Work out the finished part from the listing and answer in its coordinate system (mm). Round coordinates to 2 decimals unless told otherwise and drop trailing zeros. Order: outer loops, then holes, each group sorted by start corner. A loop starts at its lowest first (then second) coordinate and runs counter-clockwise, first axis right, second up. Notation, with made-up numbers: (21, 55) -> (43, 55) arc R22 ccw to (43, 72) -> close; hole circle Ø3 at (43.5, -2.5). An arc over 180 degrees is marked (long way). Use one line per item in the form item = value.
```python
from build123d import *

# Parameters (mm, degrees)
BOSS_EXTRUDE1_DEPTH = 3
FILLET1_R           = 10
SKETCH2_R           = 4.25
CUT_EXTRUDE1_DEPTH  = 126.335549626


with BuildPart() as part:
    # Sketch1 → Boss-Extrude1 (new body)
    with BuildSketch(Plane.XY):
        Polygon((0, 0), (0, 60), (110, 60), (110, 20), (75.358983849, 0), align=None)
    extrude(amount=BOSS_EXTRUDE1_DEPTH)

    # Fillet1
    fillet1_edges = [part.edges().sort_by_distance(p)[0] for p in [
        (110, 60, 1.5),
        (110, 20, 1.5),
        (75.358983849, 0, 1.5),
    ]]
    fillet(fillet1_edges, radius=FILLET1_R)

    # Sketch2 → Cut-Extrude1 (cut, through all)
    with BuildSketch(Plane.XY.offset(3)):
        with Locations((35, 15)):
            Circle(SKETCH2_R)
        with Locations((85, 45)):
            Circle(SKETCH2_R)
    extrude(amount=-CUT_EXTRUDE1_DEPTH, mode=Mode.SUBTRACT)


solid = part.part
```
Item 1: Consider line 1 along Y through (x, z) = (35, 0.8); line 2 along X through (y, z) = (41.5, 0.25); line 3 along Y through (x, z) = (85, 1.3). Determine where each line is inside the solid, lowest interval first.
Findings:
line_1 = 0 to 10.75, 19.25 to 60
line_2 = 0 to 82.59, 87.41 to 110
line_3 = 5.57 to 40.75, 49.25 to 60
Item 2: The part is cut by section A-A, the plane y = 45. Give the vertices of the cut face in (x, z), and give its area (4 significant figures).
Findings:
outline = (0, 0) -> (80.75, 0) -> (80.75, 3) -> (0, 3) -> close; (89.25, 0) -> (110, 0) -> (110, 3) -> (89.25, 3) -> close
area = 304.5 mm^2
Item 3: The part is cut by section C-C, the plane x = 35. Give the vertices of the cut face in (y, z).
Findings:
outline = (0, 0) -> (10.75, 0) -> (10.75, 3) -> (0, 3) -> close; (19.25, 0) -> (60, 0) -> (60, 3) -> (19.25, 3) -> close
Item 4: The part is cut by section B-B, the plane z = 2.1. Give the vertices of the cut face in (x, y), and give its area (3 significant figures).
Findings:
outline = (0, 0) -> (72.68, 0) arc R10 ccw to (77.68, 1.34) -> (105, 17.11) arc R10 ccw to (110, 25.77) -> (110, 50) arc R10 ccw to (100, 60) -> (0, 60) -> close; hole circle Ø8.5 at (35, 15); hole circle Ø8.5 at (85, 45)
area = 6,110 mm^2
Item 5: Determine the mould class of faces 1 (the cylindrical face through (108.7, 20.84, 1.52)), 2 (the cylindrical face through (30.754, 15.187, 1.521)), 3 (the flat face through (56, 30, 0)), 4 (the cylindrical face through (84.08, 40.85, 1.52)) for opening direction Y: released by +Y, released by -Y, zero draft, split by the parting line, or undercut.
Findings:
face_1 = released by -Y
face_2 = undercut
face_3 = zero draft
face_4 = undercut
Item 6: The part is cut by section D-D, the plane x = 79. Give the vertices of the cut face in (y, z), and give its area (3 significant figures).
Findings:
outline = (2.1, 0) -> (60, 0) -> (60, 3) -> (2.1, 3) -> close
area = 174 mm^2
